Build history of the part. All positions in model axes, mm. A direction names the side the tool comes from. Give positions to 0.01 mm unless a question says otherwise; leave off trailing zeros. Loops run counter-clockwise (first coordinate to the right, second up) from the corner with the lowest first, then second, coordinate; pieces in that order, holes last. Notation, with made-up numbers: (56.5, 18.25) -> (79.5, 18.25) arc R19 cw to (79.5, 30.25) -> close; hole circle Ø4 at (45.25, 8). An arc over 180 degrees is marked (long way). Answer in a Markdown table with one row per item. Add a question column.
from build123d import *

# Parameters (mm, degrees)
BOSS_EXTRUDE1_DEPTH = 3
SKETCH2_R           = 0.938992972
CUT_EXTRUDE1_DEPTH  = 0.4
BOSS_EXTRUDE2_DEPTH = 17
SKETCH5_R           = 11.578602023
CUT_EXTRUDE2_DEPTH  = 2


with BuildPart() as part:
    # Sketch1 → Boss-Extrude1 (new body)
    with BuildSketch(Plane(origin=(0, 0, 0), x_dir=(1, 0, 0), z_dir=(0, 1, 0))):
        with BuildLine():
            Line((-16.5, 14.065984754), (-15.453193913, 14.065984754))
            ThreePointArc((-15.453193913, 14.065984754), (-15.099640522, 13.919538145), (-14.953193913, 13.565984754))
            Line((-14.953193913, 13.565984754), (-14.953193913, 12.490105557))
            ThreePointArc((-14.953193913, 12.490105557), (-15.099640522, 12.136552166), (-15.453193913, 11.990105557))
            Line((-15.453193913, 11.990105557), (-16.5, 11.990105557))
            ThreePointArc((-16.5, 11.990105557), (-16.853553391, 11.843658947), (-17, 11.490105557))
            Line((-17, 11.490105557), (-17, -18))
            ThreePointArc((-17, -18), (-16.414213562, -19.414213562), (-15, -20))
            Line((-15, -20), (15, -20))
            ThreePointArc((15, -20), (16.414213562, -19.414213562), (17, -18))
            Line((17, -18), (17, 11.490105557))
            ThreePointArc((17, 11.490105557), (16.853553391, 11.843658947), (16.5, 11.990105557))
            Line((16.5, 11.990105557), (15.453193913, 11.990105557))
            ThreePointArc((15.453193913, 11.990105557), (15.099640522, 12.136552166), (14.953193913, 12.490105557))
            Line((14.953193913, 12.490105557), (14.953193913, 13.565984754))
            ThreePointArc((14.953193913, 13.565984754), (15.099640522, 13.919538145), (15.453193913, 14.065984754))
            Line((15.453193913, 14.065984754), (16.5, 14.065984754))
            ThreePointArc((16.5, 14.065984754), (16.853553391, 14.212431364), (17, 14.565984754))
            Line((17, 14.565984754), (17, 18))
            ThreePointArc((17, 18), (16.414213562, 19.414213562), (15, 20))
            Line((15, 20), (-15, 20))
            ThreePointArc((-15, 20), (-16.414213562, 19.414213562), (-17, 18))
            Line((-17, 18), (-17, 14.565984754))
            ThreePointArc((-17, 14.565984754), (-16.853553391, 14.212431364), (-16.5, 14.065984754))
        make_face()
    extrude(amount=BOSS_EXTRUDE1_DEPTH)

    # Sketch2 → Cut-Extrude1 (cut)
    with BuildSketch(Plane(origin=(0, 3, 0), x_dir=(1, 0, 0), z_dir=(0, 1, 0))):
        with Locations(Location((-15, 18, 0), (0, 0, 270))):
            Circle(SKETCH2_R)
        with Locations(Location((-15, -18, 0), (0, 0, 90))):
            Circle(SKETCH2_R)
        with Locations(Location((15, -18, 0), (0, 0, 270))):
            Circle(SKETCH2_R)
        with Locations(Location((15, 18, 0), (0, 0, 90))):
            Circle(SKETCH2_R)
    extrude(amount=-CUT_EXTRUDE1_DEPTH, mode=Mode.SUBTRACT)

    # Sketch4 → Boss-Extrude2 (add)
    with BuildSketch(Plane(origin=(0, 3, 0), x_dir=(1, 0, 0), z_dir=(0, 1, 0))):
        with BuildLine():
            Line((8.287121405, 14.483706302), (8.287121405, 20))
            Line((8.287121405, 20), (-8.287121405, 20))
            Line((-8.287121405, 20), (-8.287121405, 14.483706302))
            ThreePointArc((-8.287121405, 14.483706302), (0, -16.686944879), (8.287121405, 14.483706302))
        make_face()
    extrude(amount=BOSS_EXTRUDE2_DEPTH)

    # Sketch5 → Cut-Extrude2 (cut)
    with BuildSketch(Plane(origin=(0, 20, 0), x_dir=(1, 0, 0), z_dir=(0, 1, 0))):
        with Locations(Location((0, 0, 0), (0, 0, 270))):
            Circle(SKETCH5_R)
    extrude(amount=-CUT_EXTRUDE2_DEPTH, mode=Mode.SUBTRACT)


solid = part.part
(1) 3-axis set-ups, long thin cutter, end or side, ignore diameter. For faces 1 (the flat face through (8.287, 11, -17)), 2 (the flat face through (0, 18, 0)), 3 (the flat face through (-16, 1, -14.066)): which of +Z, -Z, +X, -X, +Y, -Y reach the whole face in a straight line?
(2) Saw through at D-D, the plane x = -6. List the corners of the cut face in (y, z), then the cut area to 3 significant figures.
(3) Wall check: line 1 along X through (y, z) = (2.8, 18); line 2 along X through (y, z) = (19.35, 0); line 3 along Y through (x, z) = (2, 17.5). Give the ranges that are in metal, low to high. Write a range as from..to.
(4) Saw through at C-C, the plane y = 4. List the corners of the cut face in (x, z), then the cut area to 3 significant figures.
(5) Saw through at A-A, the plane z = 0. List the corners of the cut face in (x, y), then the cut area to 3 significant figures.
(6) Flat gauge pins, fed straight in: pin 1 Ø6 at (x, y) = (11, 16) entering from +Z; pin 2 Ø0.5 at (y, z) = (2, -13) entering from +X; pin 3 Ø1.2 at (x, y) = (-16, 1.5) entering from -Z. Where does each tip first touch, or does it go through?
(7) Two-plate mould, pull along Z, no slides. Class faces 4 (the flat face through (-14.953, 1, -13)), 5 (the flat face through (16, 1, -14.066)), 6 (the flat face through (0, 0, 0)), 7 (the cylindrical face through (-0.612, 11.381, 16.676)): released by +Z, released by -Z, zero draft, split by the parting line, or undercut.
(8) Saw through at B-B, the plane x = 0. List the corners of the cut face in (y, z).
Worked answers:
| question | item | result |
|---|---|---|
| 1 | face 1 | -Z, +X, +Y |
| 1 | face 2 | +Y |
| 1 | face 3 | -X, +Y, -Y |
| 2 | outline | (0, -20) -> (20, -20) -> (20, -9.9) -> (18, -9.9) -> (18, 9.9) -> (20, 9.9) -> (20, 15.57) -> (3, 15.57) -> (3, 20) -> (0, 20) -> close |
| 2 | area | 685 mm^2 |
| 3 | line 1 | -17..-15.94, -14.06..14.06, 15.94..17 |
| 3 | line 2 | -16.69..-11.58, 11.58..16.69 |
| 3 | line 3 | 0..3 |
| 4 | outline | (-8.29, -20) -> (8.29, -20) -> (8.29, -14.48) arc R16.69 ccw (long way) to (-8.29, -14.48) -> close |
| 4 | area | 942 mm^2 |
| 5 | outline | (-17, 0) -> (17, 0) -> (17, 3) -> (16.69, 3) -> (16.69, 20) -> (11.58, 20) -> (11.58, 18) -> (-11.58, 18) -> (-11.58, 20) -> (-16.69, 20) -> (-16.69, 3) -> (-17, 3) -> close |
| 5 | area | 623 mm^2 |
| 6 | pin 1 | z = 14.64 |
| 6 | pin 2 | x = 14.95 |
| 6 | pin 3 | z = -19.96 |
| 7 | face 4 | undercut |
| 7 | face 5 | undercut |
| 7 | face 6 | zero draft |
| 7 | face 7 | split by the parting line |
| 8 | outline | (0, -20) -> (20, -20) -> (20, -11.58) -> (18, -11.58) -> (18, 11.58) -> (20, 11.58) -> (20, 16.69) -> (3, 16.69) -> (3, 20) -> (0, 20) -> close |
